Source: CAD feature listing. Evaluate the final solid. Frame: model axes, mm. Coordinates: 2 decimals unless noted, no trailing zeros. Order: outer loops, then holes, each group sorted by start corner. A loop starts at its lowest first (then second) coordinate and runs counter-clockwise, first axis right, second up. Notation, with made-up numbers: (-9, -30) - (43, -30) arc R33 ccw to (43, 1) - close; hole circle Ø1 at (31, 76). An arc over 180 degrees is marked (long way). One line per question, with ' | ' between items. Start each with the question number.
(1) Section C-C (y = 4). Return the cut outline in (x, z), then the cut area to 3 significant figures.
(2) Section A-A (z = -42.5). Return the cut outline in (x, y).
(3) Line query: line 1 along Y through (x, z) = (3, -30); line 2 along Y through (x, z) = (-1.75, -43.5). Output: solid intervals per line, ascending.
(4) Section B-B (x = 12). Return the cut outline in (y, z).
(5) Contact query for flat-ended pins moving along their axis: P1, Ø3, axis at x = 5.5, z = -41, coming from the -Y side; P2, Ø8, axis at x = 12, z = -18.5, coming from the -Y side; P3, Ø2, axis at x = 3.5, z = -30.5, coming from the +Y side. Output: stop coordinate, or through.
Autodesk Inventor part; units mm, degrees
ref_plane "YZ Plane" through (0, 0, 0) normal (1, 0, 0) x (0, 1, 0)
ref_plane "XZ Plane" through (0, 0, 0) normal (0, 1, 0) x (-1, 0, 0)
ref_plane "XY Plane" through (0, 0, 0) normal (0, 0, 1) x (1, 0, 0)
sketch "Szkic1" plane through (0, 0, 0) normal (0, 0, 1) x (1, 0, 0)
  circle A0 centre (3.1, 43) radius 7
  line L0 (-2, 50) -> (-2, 0)
  line L1 (-2, 50) -> (0, 50)
  line L2 (-3.9, 43) -> (-3.9, 0)
  line L3 (-3.9, 0) -> (-2, 0)
  line L4 (-3.9, 0) -> (14.8489, 5.0238)
  line L5 (-3.9, 0) -> (15.5103, 0) construction
  line L6 (1.3909, 1.4177) -> (0.8733, 3.3496)
  line L7 (0.8733, 3.3496) -> (-3.9, 2.0706)
  line L8 (0.8733, 3.3496) -> (13.2644, 6.6697)
  line L9 (13.85, 30) -> (13.85, 0)
  line L10 (13.85, 6.8267) -> (16.85, 7.6305)
  line L11 (13.85, 4.7561) -> (16.85, 5.5599)
  line L12 (16.85, 7.6305) -> (16.85, 5.5599)
  line L13 (13.85, 6.8267) -> (13.2644, 6.6697)
  point P0 (0, 0)
  point P1 (-2, 0)
  point P2 (16.85, 6.5952)
  dimension "d0" = 50
  dimension "d1" = 15
  dimension "d2" = 2
  dimension "d3" = 3
extrude "Wyciągnięcie proste1" add sketch "Szkic1" against normal blind 50 contours L7 L6 L4 L0 | L0 L4 L2 L7 | L8 L13 L9 L4 L6 | L9 L10 L12 L11 L4
properties part number "noz"
Response values:
1) outline: (3.3, -50) - (11.03, -50) - (11.03, 0) - (3.3, 0) - close | area: 386 mm²
2) outline: (-3.9, 0) - (14.85, 5.02) - (16.85, 5.56) - (16.85, 7.63) - (13.85, 6.83) - (13.26, 6.67) - (0.87, 3.35) - (-3.9, 2.07) - close
3) line 1: y = 1.85 to 3.92 | line 2: y = 0.58 to 2.65
4) outline: (4.26, -50) - (6.33, -50) - (6.33, 0) - (4.26, 0) - close
5) P1: stops at y = 2.12 | P2: stops at y = 3.19 | P3: stops at y = 4.32
